Design review of the part built by this model. Coordinates are the model's own, in mm. A direction names the side the tool comes from. Coordinates: 2 decimals unless noted, no trailing zeros. Write each loop counter-clockwise with the first axis right and the second up, starting at its lowest first coordinate (ties: lowest second). Pieces come first, ordered by that corner, then holes. Notation, with made-up numbers: (18, -15) -> (50, -15) arc R19 cw to (50, 10) -> close; hole circle Ø11 at (4, 68). An arc over 180 degrees is marked (long way). Answer in a Markdown table with one row per item. Add a question column.
Item 1: Take a section at B-B, the plane x = 0. Write out the cut boundary in (y, z).
Item 2: To check wall thickness, follow line 1 (X direction, y = 28.5, z = -7.75); line 2 (Y direction, x = 8, z = -11.5). State the ranges of each line that lie inside material, in increasing order.
Item 3: Clearance check with a flat-ended pin moving along its axis: P1, Ø14.5, axis at y = 23.85, z = 0, coming from the +X side. State where the tip first meets the part, or that it passes through.
Item 4: Take a section at C-C, the plane z = -9.25. Write out the cut boundary in (x, y), and give its area (3 significant figures).
Item 5: For faces 1 (the face through (0, 29, -11.112)), 2 (the face through (-11.9, 16.09, 1.72)), list the 3-axis set-ups (+Z, -Z, +X, -X, +Y, -Y) from which the entire face can be reached by the end or side of a thin tool; tool diameter is ignored.
Item 6: Draft analysis for pull direction X (two halves, no side actions). For faces 3 (the face through (11.92, 16.09, 1.72)), 4 (the face through (0, 29, 11.112)), 5 (the face through (-12.7, 32, -3)), state which applies: released by +X, released by -X, zero draft, split by the parting line, or undercut.
Item 7: Take a section at A-A, the plane z = 0. Write out the cut boundary in (x, y).
Item 8: Take a section at D-D, the plane y = 13.5. Write out the cut boundary in (x, z), and give its area (3 significant figures).
from build123d import *

# Parameters (mm, degrees)
SKETCH1_W           = 25.4
SKETCH1_H           = 25.4
SKETCH1_W_2         = 22.225
SKETCH1_H_2         = 22.225
BOSS_EXTRUDE1_DEPTH = 63.99895
SKETCH2_R           = 12.7
CUT_EXTRUDE1_DEPTH  = 71.016538054
SKETCH3_R           = 7.9502
CUT_EXTRUDE2_DEPTH  = 71.016538223


with BuildPart() as part:
    # Sketch1 → Boss-Extrude1 (new body)
    with BuildSketch(Plane(origin=(0, 0, 0), x_dir=(1, 0, 0), z_dir=(0, 1, 0))):
        Rectangle(SKETCH1_W, SKETCH1_H)
        Rectangle(SKETCH1_W_2, SKETCH1_H_2, mode=Mode.SUBTRACT)
    extrude(amount=BOSS_EXTRUDE1_DEPTH)

    # Sketch2 → Cut-Extrude1 (cut, through all)
    with BuildSketch(Plane.XY.offset(12.7)):
        with Locations((0, 63.998950185)):
            Circle(SKETCH2_R)
    extrude(amount=-CUT_EXTRUDE1_DEPTH, mode=Mode.SUBTRACT)

    # Sketch3 → Cut-Extrude2 (cut, through all)
    with BuildSketch(Plane(origin=(12.7, 0, 0), x_dir=(0, 0, -1), z_dir=(1, 0, 0))):
        with Locations((0, 23.8506)):
            Circle(SKETCH3_R)
    extrude(amount=-CUT_EXTRUDE2_DEPTH, mode=Mode.SUBTRACT)


solid = part.part
Answers:
| question | item | result |
|---|---|---|
| 1 | outline | (0, -12.7) -> (51.3, -12.7) -> (51.3, -11.11) -> (0, -11.11) -> close; (0, 11.11) -> (51.3, 11.11) -> (51.3, 12.7) -> (0, 12.7) -> close |
| 2 | line 1 | x = -12.7 to -11.11, 11.11 to 12.7 |
| 2 | line 2 | y = 0 to 54.14 |
| 3 | P1 | passes through |
| 4 | outline | (-12.7, 0) -> (-11.11, 0) -> (-11.11, 57.85) arc R12.7 cw to (-12.7, 64) -> close; (11.11, 0) -> (12.7, 0) -> (12.7, 64) arc R12.7 cw to (11.11, 57.85) -> close |
| 4 | area | 190 mm^2 |
| 5 | face 1 | +Y, -Y |
| 5 | face 2 | +X, -X |
| 6 | face 3 | zero draft |
| 6 | face 4 | undercut |
| 6 | face 5 | released by -X |
| 7 | outline | (-12.7, 0) -> (-11.11, 0) -> (-11.11, 15.9) -> (-12.7, 15.9) -> close; (-12.7, 31.8) -> (-11.11, 31.8) -> (-11.11, 57.85) arc R12.7 cw to (-12.7, 64) -> close; (11.11, 0) -> (12.7, 0) -> (12.7, 15.9) -> (11.11, 15.9) -> close; (11.11, 31.8) -> (12.7, 31.8) -> (12.7, 64) arc R12.7 cw to (11.11, 57.85) -> close |
| 8 | outline | (-12.7, -12.7) -> (12.7, -12.7) -> (12.7, 12.7) -> (-12.7, 12.7) -> close; hole (-11.11, -11.11) -> (11.11, -11.11) -> (11.11, 11.11) -> (-11.11, 11.11) -> close |
| 8 | area | 151 mm^2 |
